Verification items for the finished model (mm, model axes). Face numbers are marked on the shaded views. A direction names the side the tool comes from. Round coordinates to 2 decimals unless told otherwise and drop trailing zeros. Write each loop counter-clockwise with the first axis right and the second up, starting at its lowest first coordinate (ties: lowest second). Pieces come first, ordered by that corner, then holes. Notation, with made-up numbers: M 71,59.5 L 102,59.5 A9 cw 102,74.5 Z; hole C 5.25,-16.5 d5. An arc over 180 degrees is marked long. Write each question's results on one line, items separated by ' | '.
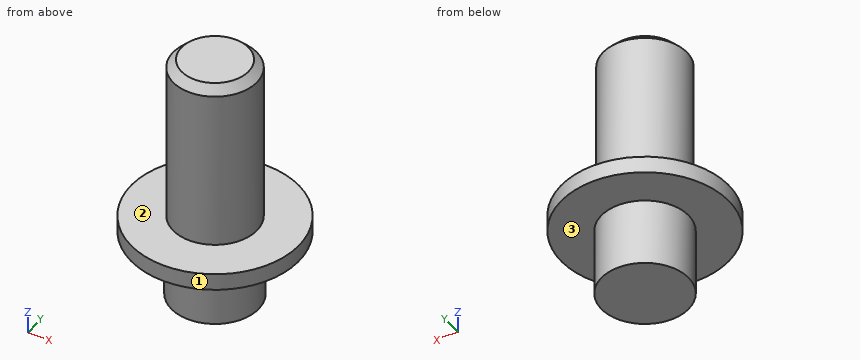
Autodesk Inventor part; units mm, degrees
ref_plane "YZ Plane" through (0, 0, 0) normal (1, 0, 0) x (0, 1, 0)
ref_plane "XZ Plane" through (0, 0, 0) normal (0, 1, 0) x (-1, 0, 0)
ref_plane "XY Plane" through (0, 0, 0) normal (0, 0, 1) x (1, 0, 0)
sketch "Sketch1" plane through (0, 0, 0) normal (0, 0, 1) x (1, 0, 0)
  circle A0 centre (0, 0) radius 6.35
  dimension "d0" = 12.7
extrude "Extrusion1" add sketch "Sketch1" along normal blind 1.27
sketch "Sketch2" plane through (0, 0, 1.27) normal (0, 0, 1) x (1, 0, 0)
  circle A0 centre (0, 0) radius 6.35
  circle A1 centre (0, 0) radius 3.175
  dimension "d3" = 6.35
extrude "Extrusion2" add sketch "Sketch2" along normal blind 12.7 contours A1
chamfer "Chamfer1" distance 0.635 angle 45 1 edges at (-3.175, 0, 13.97)
thread "Thread1"
sketch "Sketch3" plane through (0, 0, 0) normal (0, 0, -1) x (-1, 0, 0)
  circle A0 centre (0, 0) radius 6.35
  circle A1 centre (0, 0) radius 3.302
  dimension "d10" = 6.604
extrude "Extrusion3" add sketch "Sketch3" along normal blind 5.08 contours A1
properties part number "Breaker Post" material "Steel, Mild"
1) Sectioned sample at A-A, the plane x = 0. Record the cut outline in (y, z) (3 decimals).
Calculated:
outline: M -6.35,0 L -3.302,0 L -3.302,-5.08 L 3.302,-5.08 L 3.302,0 L 6.35,0 L 6.35,1.27 L 3.175,1.27 L 3.175,13.335 L 2.54,13.97 L -2.54,13.97 L -3.175,13.335 L -3.175,1.27 L -6.35,1.27 Z
2) Sectioned sample at D-D, the plane y = 4. Record the cut outline in (x, z).
Calculated:
outline: M -4.93,0 L 4.93,0 L 4.93,1.27 L -4.93,1.27 Z
3) Access from +Z, -Z, +X, -X, +Y, -Y to the whole of each face (thin tool, end or side, straight path). Record for the marked faces 1, 2 and 3.
Calculated:
face 1: +Z, -Z | face 2: +Z | face 3: -Z
4) Sectioned sample at C-C, the plane z = 3.75. Record the cut outline in (x, y) (3 decimals).
Calculated:
outline: C 0,0 d6.35
5) Material ranges on line 1 (Z direction, x = 0.75, y = 5.5); line 2 (X direction, y = 5.5, z = 1); line 3 (X direction, y = 1.75, z = 7.5), recorded low to high. Write a range as [from, to].
Calculated:
line 1: z = [0, 1.27] | line 2: x = [-3.17, 3.17] | line 3: x = [-2.65, 2.65]
6) Depth check by flat-ended pin: P1, Ø2, axis at x = 1, z = 5.5, coming from the -Y side (3 decimals); P2, Ø4, axis at y = -3, z = 7, coming from the -X side. Enter the tip coordinate at first touch or a pass-through.
Calculated:
P1: stops at y = -3.175 | P2: stops at x = -3.01
